```python
from build123d import *

# Parameters (mm, degrees)
EXTRUDE_1_DEPTH          = 100
SKETCH_2_R               = 30
CUT_EXTRUDE_1_DEPTH      = 100
SKETCH_3_R               = 32.5
SKETCH_3_R_2             = 30
EXTRUDE_2_DEPTH          = 5
EXTRUDE_START            = 5
SKETCH_4_R               = 32.5
SKETCH_4_R_2             = 30
EXTRUDE_3_DEPTH          = 5
SKETCH_5_R               = 30
CUT_EXTRUDE_2_DEPTH      = 248
SKETCH_6_R               = 35
SKETCH_6_R_2             = 30
EXTRUDE_4_DEPTH          = 5
SKETCH_7_R               = 35
SKETCH_7_R_2             = 30
EXTRUDE_5_DEPTH          = 5
SKETCH_8_R               = 60
EXTRUDE_6_DEPTH          = 558
SKETCH_9_R               = 60
EXTRUDE_7_DEPTH          = 1116
SKETCH_12_R              = 30
EXTRUDE_9_DEPTH          = 10
PATTERN_LINEAR_2_COUNT   = 2
PATTERN_LINEAR_2_PITCH   = 80
MIRROR_3_COPY_1_SKETCH_R = 30
MIRROR_3_COPY_1_DEPTH    = 10
SCALE1_SCALE             = 0.345


with BuildPart() as part:
    # 草图1 → 凸台-拉伸1 (new body)
    with BuildSketch(Plane.XY):
        with BuildLine():
            Line((-60.1323511, -127.533248731), (739.8676489, -277.533248731))
            Line((739.8676489, -277.533248731), (4439.8676489, -277.533248731))
            ThreePointArc((4439.8676489, -277.533248731), (4514.8676489, -202.533248731), (4439.8676489, -127.533248731))
            Line((4439.8676489, -127.533248731), (3639.8676489, 22.466751269))
            Line((3639.8676489, 22.466751269), (-60.1323511, 22.466751269))
            ThreePointArc((-60.1323511, 22.466751269), (-135.1323511, -52.533248731), (-60.1323511, -127.533248731))
        make_face()
    extrude(amount=EXTRUDE_1_DEPTH)

    # 草图2 → 切除-拉伸1 (cut)
    with BuildSketch(Plane.XY.offset(100)):
        with Locations((-60.1323511, -52.533248731)):
            Circle(SKETCH_2_R)
        with Locations((4439.8676489, -202.533248731)):
            Circle(SKETCH_2_R)
    extrude(amount=-CUT_EXTRUDE_1_DEPTH, mode=Mode.SUBTRACT)

    # 草图3 → 凸台-拉伸2 (add)
    # profile 1 of 2: a face of its own
    with BuildSketch(Plane(origin=(0, 0, 0), x_dir=(-1, 0, 0), z_dir=(0, 0, -1))):
        with Locations(Location((-4439.8676489, -202.533248731, 0), (0, 0, 180))):
            Circle(SKETCH_3_R)
        with Locations(Location((-4439.8676489, -202.533248731, 0), (0, 0, 180))):
            Circle(SKETCH_3_R_2, mode=Mode.SUBTRACT)
    # profile 2 of 2: a face of its own
    with BuildSketch(Plane(origin=(0, 0, 0), x_dir=(-1, 0, 0), z_dir=(0, 0, -1))):
        with Locations(Location((60.1323511, -52.533248731, 0), (0, 0, 180))):
            Circle(SKETCH_3_R)
        with Locations(Location((60.1323511, -52.533248731, 0), (0, 0, 180))):
            Circle(SKETCH_3_R_2, mode=Mode.SUBTRACT)
    extrude(amount=EXTRUDE_2_DEPTH)

    # 草图4 → 凸台-拉伸3 (add)
    # profile 1 of 2: a face of its own
    with BuildSketch(Plane.XY.offset(100).offset(EXTRUDE_START)):
        with Locations((-60.1323511, -52.533248731)):
            Circle(SKETCH_4_R)
        with Locations((-60.1323511, -52.533248731)):
            Circle(SKETCH_4_R_2, mode=Mode.SUBTRACT)
    # profile 2 of 2: a face of its own
    with BuildSketch(Plane.XY.offset(100).offset(EXTRUDE_START)):
        with Locations((4439.8676489, -202.533248731)):
            Circle(SKETCH_4_R)
        with Locations((4439.8676489, -202.533248731)):
            Circle(SKETCH_4_R_2, mode=Mode.SUBTRACT)
    extrude(amount=-EXTRUDE_3_DEPTH)

    # 草图5 → 切除-拉伸2 (cut)
    with BuildSketch(Plane(origin=(0, 0, 0), x_dir=(-1, 0, 0), z_dir=(0, 0, -1))):
        with Locations((-2189.8676489, -127.533248731)):
            Circle(SKETCH_5_R)
    extrude(amount=-CUT_EXTRUDE_2_DEPTH, mode=Mode.SUBTRACT)

    # 草图6 → 凸台-拉伸4 (add)
    with BuildSketch(Plane(origin=(0, 0, 0), x_dir=(-1, 0, 0), z_dir=(0, 0, -1)).offset(EXTRUDE_START)):
        with Locations(Location((-2189.8676489, -127.533248731, 0), (0, 0, 180))):
            Circle(SKETCH_6_R)
        with Locations((-2189.8676489, -127.533248731)):
            Circle(SKETCH_6_R_2, mode=Mode.SUBTRACT)
    extrude(amount=-EXTRUDE_4_DEPTH)

    # 草图7 → 凸台-拉伸5 (add)
    with BuildSketch(Plane.XY.offset(100)):
        with Locations((2189.8676489, -127.533248731)):
            Circle(SKETCH_7_R)
        with Locations(Location((2189.8676489, -127.533248731, 0), (0, 0, 180))):
            Circle(SKETCH_7_R_2, mode=Mode.SUBTRACT)
    extrude(amount=EXTRUDE_5_DEPTH)

    # 草图8 → 凸台-拉伸6 (add)
    with BuildSketch(Plane.XY.offset(100)):
        with Locations((739.8676489, -127.533248731)):
            Circle(SKETCH_8_R)
    extrude(amount=EXTRUDE_6_DEPTH)

    # 镜向1: part across plane


with BuildPart() as part_1:
    add(part.part)
    add(part.part.mirror(Plane(origin=(739.8676489, -127.533248731, 658), x_dir=(1, 0, 0), z_dir=(0, 0, 1))))

    # 草图9 → 凸台-拉伸7 (add)
    with BuildSketch(Plane(origin=(0, 0, 1216), x_dir=(-1, 0, 0), z_dir=(0, 0, -1))):
        with Locations(Location((-3939.8676489, -157.533248731, 0), (0, 0, 180))):
            Circle(SKETCH_9_R)
    extrude(amount=EXTRUDE_7_DEPTH)

    # 草图12 → 凸台-拉伸9 (add)
    with BuildSketch(Plane(origin=(0, 0, 370), x_dir=(-1, 0, 0), z_dir=(0, 0, -1))):
        with BuildLine():
            Line((-3730.655081085, -184.553638593), (-3908.372573379, -95.018768665))
            ThreePointArc((-3908.372573379, -95.018768665), (-4005.218278755, -132.447492263), (-3958.292598451, -225.06488009))
            Line((-3958.292598451, -225.06488009), (-3766.312241851, -277.443718182))
            ThreePointArc((-3766.312241851, -277.443718182), (-3706.472542276, -247.125236117), (-3730.655081085, -184.553638593))
        make_face()
        with Locations((-3753.151563601, -229.20683864)):
            Circle(SKETCH_12_R, mode=Mode.SUBTRACT)
    extrude_9 = extrude(amount=EXTRUDE_9_DEPTH)

    # 阵列(线性)2: 凸台-拉伸9 ×2
    with Locations(*[(0, 0, -i * PATTERN_LINEAR_2_PITCH) for i in range(1, PATTERN_LINEAR_2_COUNT)]):
        add(extrude_9)

    # 镜向3: 凸台-拉伸9 across plane
    add(extrude_9.mirror(Plane(origin=(0, 0, 658), x_dir=(1, 0, 0), z_dir=(0, 0, -1))))

    # 镜向3 copy 1 sketch → 镜向3 copy 1 (add)
    with BuildSketch(Plane(origin=(0, 0, 1026), x_dir=(-1, 0, 0), z_dir=(0, 0, 1))):
        with BuildLine():
            Line((-3730.655081085, 184.553638593), (-3908.372573379, 95.018768665))
            ThreePointArc((-3908.372573379, 95.018768665), (-4005.218278755, 132.447492263), (-3958.292598451, 225.06488009))
            Line((-3958.292598451, 225.06488009), (-3766.312241851, 277.443718182))
            ThreePointArc((-3766.312241851, 277.443718182), (-3706.472542276, 247.125236117), (-3730.655081085, 184.553638593))
        make_face()
        with Locations((-3753.151563601, 229.20683864)):
            Circle(MIRROR_3_COPY_1_SKETCH_R, mode=Mode.SUBTRACT)
    extrude(amount=MIRROR_3_COPY_1_DEPTH)


with BuildPart() as part_2:
    # Scale1: scaled about (2208.887322041, -129.132987592, 658)
    add(part_1.part.scale(SCALE1_SCALE).moved(Location((1446.821195937, -84.582106873, 430.99))))


solid = part_2.part
```
Can you work these out from the model? Positions are in its coordinate system, mm. A direction names the side the tool comes from. Round coordinates to 2 decimals unless told otherwise and drop trailing zeros. Loops run counter-clockwise (first coordinate to the right, second up) from the corner with the lowest first, then second, coordinate; pieces in that order, holes last. Notation, with made-up numbers: (34, 18) -> (81, 18) arc R29 ccw to (81, 45) -> close; hole circle Ø11 at (7, 71). An arc over 180 degrees is marked (long way). Answer in a Markdown table with one row per item.
Item 1: Suppose I cut it at B-B, the plane z = 704. List the corners of the cut face in (x, y) for me, plus the area to 3 significant figures.
Answer block:
| item | result |
|---|---|
| outline | circle Ø41.4 at (1702.08, -128.58); circle Ø41.4 at (2806.08, -138.93) |
| area | 2,690 mm² |
Item 2: If I drill on probe 1 along Z at (x, y) = (2762, -164); probe 2 along Z at (x, y) = (2883.5, -174.5); probe 3 along X at (y, z) = (-128, 836.5), over which ranges is the centre line in solid material (lowest first)?
Answer block:
| item | result |
|---|---|
| probe 1 | 430.99 to 465.49, 527.59 to 531.04, 555.19 to 558.64, 757.36 to 760.81, 784.96 to 788.41, 850.51 to 885.01 |
| probe 2 | 430.99 to 465.49, 850.51 to 885.01 |
| probe 3 | 1681.38 to 1722.77, 2788.5 to 2823.65 |
Item 3: Will these pins go through, and if not, where does the flat tip stop? P1, Ø1, axis at x = 1855.5, y = -108, coming from the +Z side; P2, Ø10.5, axis at x = 2510, z = 453, coming from the -Y side; P3, Ø18.5, axis at x = 1426.08, y = -102.71, coming from the -Z side; P4, Ø2, axis at y = -147, z = 515.5, coming from the +X side.
Answer block:
| item | result |
|---|---|
| P1 | z = 885.01 |
| P2 | y = -180.33 |
| P3 | through |
| P4 | x = 2825.53 |
Item 4: We'd pull the mould along X, two halves only. Please class faces 1 (the cylindrical face through (1400.207, -102.137, 447.999)), 2 (the flat face through (2766, -155, 760.81)), 3 (the cylindrical face through (3004.444, -155.025, 447.999)), 4 (the flat face through (2331, -180.331, 448)): released by +X, released by -X, zero draft, split by the parting line, or undercut.
Answer block:
| item | result |
|---|---|
| face 1 | released by -X |
| face 2 | undercut |
| face 3 | released by +X |
| face 4 | zero draft |
Item 5: On a 3-axis mill with a long thin cutter (end or side, diameter ignored), from which of +Z, -Z, +X, -X, +Y, -Y can I reach the whole of each face in a straight line? I mean faces 5 (the flat face through (2764.124, -133.025, 556.939)), 6 (the flat face through (2073, -76.831, 448)), 7 (the cylindrical face through (2825.197, -131.003, 819.895)). Say none if no direction works.
Answer block:
| item | result |
|---|---|
| face 5 | +Y |
| face 6 | +Z, -Z, +X, -X, +Y |
| face 7 | none |
Item 6: Suppose I cut it at A-A, the plane x = 1635. List the corners of the cut face in (y, z) for me.
Answer block:
| item | result |
|---|---|
| outline | (-167.75, 430.99) -> (-76.83, 430.99) -> (-76.83, 465.49) -> (-167.75, 465.49) -> close; (-167.75, 850.51) -> (-76.83, 850.51) -> (-76.83, 885.01) -> (-167.75, 885.01) -> close |
